Build history of the part. All positions in model axes, mm. Face numbers are marked on the shaded views. A direction names the side the tool comes from. Coordinates: 2 decimals unless noted, no trailing zeros. Write each loop counter-clockwise with the first axis right and the second up, starting at its lowest first coordinate (ties: lowest second). Pieces come first, ordered by that corner, then holes.
from build123d import *

# Parameters (mm, degrees)
SKETCH2_R          = 3.4925
CUT_EXTRUDE1_DEPTH = 53.937829102
SKETCH3_R          = 1.5875
CUT_EXTRUDE2_DEPTH = 54.529596078
CIRPATTERN1_COUNT  = 5
FILLET1_R          = 0.79375


with BuildPart() as part:
    # Sketch1 → Revolve1 (revolve)
    with BuildSketch(Plane.XY, mode=Mode.PRIVATE) as revolve1_sk:
        Polygon((19.33575, -14.2875), (19.33575, 0), (0, 0), (0, 4.7625), (19.33575, 4.7625), (19.33575, 9.525), (22.225, 9.525), (22.225, 4.7625), (26.9875, 4.7625), (26.9875, 6.35), (34.925, 6.35), (34.925, 0), (22.51075, 0), (22.51075, -14.2875), align=None)
    revolve(revolve1_sk.sketch.rotate(Axis((0, 0, 0), (0, 1, 0)), 90), axis=Axis((0, 0, 0), (0, 1, 0)))

    # Sketch2 → Cut-Extrude1 (cut, through all)
    with BuildSketch(Plane(origin=(0, 4.7625, 0), x_dir=(1, 0, 0), z_dir=(0, 1, 0))):
        with Locations(Location((-13.4874, 0, 0), (0, 0, 270))):
            Circle(SKETCH2_R)
        with Locations(Location((0, 13.4874, 0), (0, 0, 270))):
            Circle(SKETCH2_R)
        with Locations(Location((13.4874, 0, 0), (0, 0, 270))):
            Circle(SKETCH2_R)
        with Locations(Location((0, -13.4874, 0), (0, 0, 270))):
            Circle(SKETCH2_R)
    extrude(amount=-CUT_EXTRUDE1_DEPTH, mode=Mode.SUBTRACT)

    # Sketch3 → Cut-Extrude2 (cut, through all)
    with BuildSketch(Plane(origin=(0, 6.35, 0), x_dir=(1, 0, 0), z_dir=(0, 1, 0))):
        with Locations(Location((0, 30.95625, 0), (0, 0, 270))):
            Circle(SKETCH3_R)
    cut_extrude2 = extrude(amount=-CUT_EXTRUDE2_DEPTH, mode=Mode.SUBTRACT)

    # CirPattern1: Cut-Extrude2 ×5 about axis
    cirpattern1_axis = Axis((0, 0, 0), (0, 1, 0))
    for i in range(1, CIRPATTERN1_COUNT):
        add(cut_extrude2.rotate(cirpattern1_axis, i * 360 / CIRPATTERN1_COUNT), mode=Mode.SUBTRACT)

    # Fillet1
    fillet1_edges = [part.edges().sort_by_distance(p)[0] for p in [
        (0, 4.7625, 26.9875),
        (0, 4.7625, 22.225),
        (0, 4.7625, 19.33575),
        (0, 0, 19.33575),
    ]]
    fillet(fillet1_edges, radius=FILLET1_R)


solid = part.part
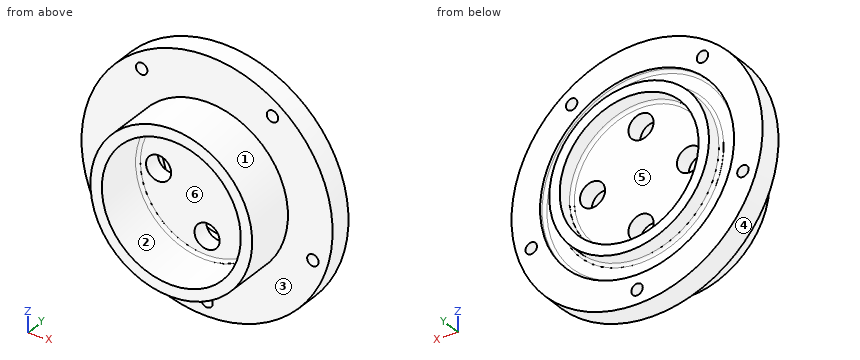
(1) Two-plate mould, pull along Z, no slides. Class the marked faces 1, 2 and 3: pulls with the +Z half, pulls with the -Z half, needs draft (parallel to the pull), parting line crosses it, or undercut.
(2) Flat gauge pins, fed straight in: P1, Ø5, axis at x = -5.5, z = 9, coming from the +Y side; P2, Ø5, axis at x = 0, z = -30.96, coming from the +Y side; P3, Ø1.5, axis at x = 14, y = -5, coming from the -Z side. Where does each tip first touch, or does it go through?
(3) Slice it at D-D, the plane y = -7.75. List the corners of the cut face in (x, z).
(4) 3-axis set-ups, long thin cutter, end or side, ignore diameter. For the marked faces 4, 5 and 6: which of +Z, -Z, +X, -X, +Y, -Y reach the whole face in a straight line?
(5) Probe L1, parallel to Y at x = -13, z = -5; L2, parallel to X at y = -6, z = 0; L3, parallel to Y at x = 23, z = -26. List the from-to ranges inside material, lowest first.
(6) Slice it at B-B, the plane x = 0. Give the number of separate pieces and of enclosed holes in the cut face, and give its area (3 significant figures).
Results:
1. face 1: parting line crosses it
1. face 2: undercut
1. face 3: needs draft
2. P1: stops at y = 4.76
2. P2: stops at y = 6.35
2. P3: stops at z = -18.2
3. outline: circle Ø45.02 at (0, 0); hole circle Ø38.67 at (0, 0)
4. face 4: +Y, -Y
4. face 5: +Y
4. face 6: -Y
5. L1: y = 0 to 4.76
5. L2: x = -22.51 to -19.34, 19.34 to 22.51
5. L3: y = 0 to 6.35
6. separate pieces: 4
6. enclosed holes: 0
6. area: 390 mm2
